```python
from build123d import *

# Parameters (mm, degrees)
CUT_EXTRUDE_1_REACH      = 37
SKETCH_2_R               = 8.25
SKETCH_3_W               = 8
SKETCH_3_H               = 6
CUT_EXTRUDE_2_DEPTH      = 35.738958199
PATTERN_CIRCULAR_1_COUNT = 4


with BuildPart() as part:
    # 草图1 → 旋转1 (revolve)
    with BuildSketch(Plane(origin=(0, 0, 0), x_dir=(1, 0, 0), z_dir=(0, 1, 0))):
        Polygon((-22, 0), (0, 0), (0, 9), (-15.698132156, 9), (-25.161358247, 35), (-34.738958199, 35), align=None)
    revolve(axis=Axis((0, 0, 0), (0, 0, -1)))

    # 草图2 → 切除-拉伸1 (cut, up to next)
    with BuildSketch(Plane.XY, mode=Mode.PRIVATE) as cut_extrude_1_sk1:
        Circle(SKETCH_2_R)
    cut_extrude_1_tool1 = extrude(cut_extrude_1_sk1.sketch, amount=-CUT_EXTRUDE_1_REACH, mode=Mode.PRIVATE) & part.part
    add(cut_extrude_1_tool1.solids().sort_by_distance((0, 0, 0))[0], mode=Mode.SUBTRACT)

    # 草图3 → 切除-拉伸2 (cut, symmetric)
    with BuildSketch(Plane(origin=(0, 0, 0), x_dir=(1, 0, 0), z_dir=(0, 1, 0))):
        with Locations((0, 32)):
            Rectangle(SKETCH_3_W, SKETCH_3_H)
    cut_extrude_2 = extrude(amount=CUT_EXTRUDE_2_DEPTH, both=True, mode=Mode.SUBTRACT)

    # 阵列(圆周)1: 切除-拉伸2 ×4 about axis
    pattern_circular_1_axis = Axis((0, 0, 0), (0, 0, 1))
    for i in range(1, PATTERN_CIRCULAR_1_COUNT):
        add(cut_extrude_2.rotate(pattern_circular_1_axis, i * 360 / PATTERN_CIRCULAR_1_COUNT), mode=Mode.SUBTRACT)


solid = part.part
```
Can you work these out from the model? Positions are in its coordinate system, mm. A direction names the side the tool comes from. Round coordinates to 2 decimals unless told otherwise and drop trailing zeros. Loops run counter-clockwise (first coordinate to the right, second up) from the corner with the lowest first, then second, coordinate; pieces in that order, holes last. Notation, with made-up numbers: (65.5, -10.5) -> (122.5, -10.5) arc R24 cw to (122.5, 0.5) -> close; hole circle Ø7 at (-26, 20.5). An arc over 180 degrees is marked (long way). One line per item, written item: value. Start each with the question number.
1. If I drill on probe 1 along Z at (x, y) = (5, 8.5); probe 2 along Y at (x, z) = (0, -3); probe 3 along Y at (x, z) = (0, -3.5), over which ranges is the centre line in solid material (lowest first)?
2. For faces 4 (the flat face through (7, -7, -9)), 5 (the flat face through (-19, -19, -35)), 6 (the flat face through (0, 28, -29)), 7 (the flat face through (28, 4, -32)), which set-ups out of +Z, -Z, +X, -X, +Y, -Y let a thin tool reach every point of the face, with its end or its side?
3. If we mould it in two halves opening along X, with no side actions, what happens to faces 1 (the flat face through (19, -19, -35)), 2 (the flat face through (4, -28, -32)), 3 (the flat face through (-4, 29, -32))? For each: pulls with the +X half, pulls with the -X half, needs draft (parallel to the pull), parting line crosses it, or undercut.
4. If we section it at C-C, the plane z = -31: Write out the boundary of the cut face in (x, y).
5. If we section it at A-A, the plane x = 0: Write out the boundary of the cut face in (y, z), then the cut area to 3 significant figures.
6. For pin 1 (3 mm diameter, centred on x = 31.5, z = -31.5, fed in from +Y); pin 2 (3 mm diameter, centred on y = -17, z = -25.5, fed in from +X); pin 3 (8 mm diameter, centred on x = -27, z = -21.5, fed in from -Y), each with a flat end and sliding along its axis, tell me the tip position at first contact or that it passes through.
Calculated:
1. probe 1: z = -9 to 0
1. probe 2: y = -23.09 to -8.25, 8.25 to 23.09
1. probe 3: y = -23.27 to -8.25, 8.25 to 23.27
2. face 4: -Z
2. face 5: -Z, +X, -X, +Y, -Y
2. face 6: -Z, +Y, -Y
2. face 7: -Z, +X, -X
3. face 1: needs draft
3. face 2: undercut
3. face 3: undercut
4. outline: (-33.04, -4) arc R33.28 ccw to (-4, -33.04) -> (-4, -23.37) arc R23.71 cw to (-23.37, -4) -> close; (-33.04, 4) -> (-23.37, 4) arc R23.71 cw to (-4, 23.37) -> (-4, 33.04) arc R33.28 ccw to start; (4, -33.04) arc R33.28 ccw to (33.04, -4) -> (23.37, -4) arc R23.71 cw to (4, -23.37) -> close; (4, 23.37) arc R23.71 cw to (23.37, 4) -> (33.04, 4) arc R33.28 ccw to (4, 33.04) -> close
5. outline: (-32.56, -29) -> (-22.98, -29) -> (-15.7, -9) -> (-8.25, -9) -> (-8.25, 0) -> (-22, 0) -> close; (8.25, -9) -> (15.7, -9) -> (22.98, -29) -> (32.56, -29) -> (22, 0) -> (8.25, 0) -> close
5. area: 660 mm²
6. pin 1: stops at y = 15.07
6. pin 2: stops at x = 27.38
6. pin 3: stops at y = -19.5
